Autodesk Inventor part; units mm, degrees
ref_plane "YZ Plane" through (0, 0, 0) normal (1, 0, 0) x (0, 1, 0)
ref_plane "XZ Plane" through (0, 0, 0) normal (0, 1, 0) x (-1, 0, 0)
ref_plane "XY Plane" through (0, 0, 0) normal (0, 0, 1) x (1, 0, 0)
sketch "Sketch1" plane through (0, 0, 0) normal (0, 1, 0) x (-1, 0, 0)
  line L0 (0, 0) -> (76.2, 0)
  line L1 (76.2, 0) -> (76.2, -25.4)
  line L2 (76.2, -25.4) -> (50.8, -25.4)
  line L3 (50.8, -25.4) -> (50.8, -50.8)
  line L4 (50.8, -50.8) -> (0, -50.8)
  line L5 (0, -50.8) -> (0, 0)
  dimension "d0" = 76.2
  dimension "d1" = 25.4
  dimension "d2" = 25.4
  dimension "d3" = 25.4
  dimension "d4" = 50.8
extrude "Extrusion1" add sketch "Sketch1" along normal blind 25.4
sketch "Sketch2" plane through (0, 25.4, 0) normal (0, 1, 0) x (1, 0, 0)
  line L0 (-50.8, 25.4) -> (-25.4, 25.4)
  line L1 (-25.4, 25.4) -> (-25.4, 50.8)
  line L2 (-25.4, 50.8) -> (-50.8, 50.8)
  line L3 (-50.8, 50.8) -> (-50.8, 25.4)
  line L4 (-50.8, 50.8) -> (-50.8, 25.4)
  point P0 (0, 0)
  dimension "d7" = 25.4
extrude "Extrusion2" add sketch "Sketch2" along normal blind 25.4
properties part number "BluePuzzlePiece"
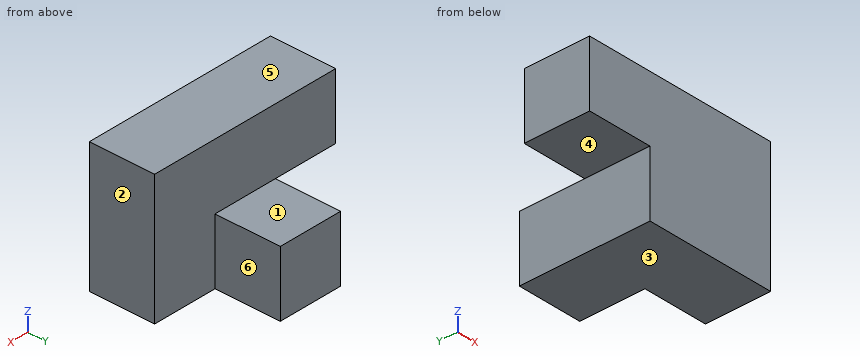
Part model, mm, in its own coordinate system. Face numbers are marked on the shaded views. A direction names the side the tool comes from. Coordinates: 2 decimals unless noted, no trailing zeros. Write each loop counter-clockwise with the first axis right and the second up, starting at its lowest first coordinate (ties: lowest second). Pieces come first, ordered by that corner, then holes.
Item 1: Slice it at B-B (x = -41.5). Write the cut outline in (y, z).
Item 2: Mould opens along Z. For the marked faces 1, 2 and 3 say: released by +Z, released by -Z, zero draft, split by the parting line, or undercut.
Item 3: Pin check, flat tips, straight feed: pin 1 (1 mm diameter, centred on x = -42, y = 30.5, fed in from +Z); pin 2 (12.5 mm diameter, centred on y = 33, z = -39.5, fed in from +X); pin 3 (8 mm diameter, centred on y = 45.5, z = -19.5, fed in from +X) (1 decimal); pin 4 (4 mm diameter, centred on y = 34.5, z = -37.5, fed in from -X). Stop position of each tip, or through.
Item 4: Which spindle directions (+Z, -Z, +X, -X, +Y, -Y) get a long thin tool onto all of the face, cutting with end or side? Do the marked faces 4, 5 and 6. Say none if no direction does.
Item 5: Slice it at A-A (y = 12). Write the cut outline in (x, z), and give its area (3 significant figures).
Item 6: Slice it at D-D (x = -64.5). Write the cut outline in (y, z).
Item 7: Slice it at C-C (z = -4). Write the cut outline in (x, y).
Item 8: Probe line 1 (Y direction, x = -56, z = -22.5); line 2 (X direction, y = 24, z = -44.5); line 3 (Z direction, x = -38, y = 34). List the from-to ranges inside material, lowest first.
Results found:
1. outline: (0, -50.8) - (50.8, -50.8) - (50.8, -25.4) - (25.4, -25.4) - (25.4, 0) - (0, 0) - close
2. face 1: released by +Z
2. face 2: zero draft
2. face 3: released by -Z
3. pin 1: stops at z = -25.4
3. pin 2: stops at x = -25.4
3. pin 3: passes through
3. pin 4: stops at x = -50.8
4. face 4: -Z, -X, +Y, -Y
4. face 5: +Z, +X, -X, +Y, -Y
4. face 6: +Z, -Z, +X, +Y
5. outline: (-76.2, -25.4) - (-50.8, -25.4) - (-50.8, -50.8) - (0, -50.8) - (0, 0) - (-76.2, 0) - close
5. area: 3,230 mm2
6. outline: (0, -25.4) - (25.4, -25.4) - (25.4, 0) - (0, 0) - close
7. outline: (-76.2, 0) - (0, 0) - (0, 25.4) - (-76.2, 25.4) - close
8. line 1: y = 0 to 25.4
8. line 2: x = -50.8 to 0
8. line 3: z = -50.8 to -25.4
